Can you work these out from the model? Positions are in its coordinate system, mm. Face numbers are marked on the shaded views. A direction names the side the tool comes from. Round coordinates to 2 decimals unless told otherwise and drop trailing zeros. Write each loop counter-clockwise with the first axis right and the second up, starting at its lowest first coordinate (ties: lowest second). Pieces come first, ordered by that corner, then holes. Notation, with made-up numbers: M 1,4 L 13,4 A34 ccw 13,36 Z; hole C -27,42.5 d9. An arc over 180 degrees is marked long. Answer in a Markdown table with one row per item. Add a question column.
(1) Suppose I cut it at A-A, the plane x = 2.5. Write out the boundary of the cut face in (y, z), then the cut area to 3 significant figures.
(2) I'm going to push flat-ended pins straight in: pin 1 (3 mm diameter, centred on y = -5, z = 4.5, fed in from +X); pin 2 (3 mm diameter, centred on x = 0, y = 0, fed in from +Z); pin 3 (3 mm diameter, centred on y = 7, z = 4.5, fed in from +X). Where does each tip first touch, or does it pass through?
(3) If we mould it in two halves opening along Y, with no side actions, what happens to the marked faces 5, 6 and 7? For each: released by +Y, released by -Y, zero draft, split by the parting line, or undercut.
(4) If I drill on probe 1 along Y at (x, z) = (0, 7.4); probe 2 along Y at (x, z) = (-12, 7); probe 3 along X at (y, z) = (10.25, 6), over which ranges is the centre line in solid material (lowest first)?
(5) Suppose I cut it at B-B, the plane x = -8.75. Write out the boundary of the cut face in (y, z), then the cut area to 3 significant figures.
(6) For the marked faces 1, 2, 3 and 4, which set-ups out of +Z, -Z, +X, -X, +Y, -Y let a thin tool reach every point of the face, with its end or its side?
(7) Suppose I cut it at C-C, the plane x = 9. Write out the boundary of the cut face in (y, z).
from build123d import *

# Parameters (mm, degrees)
BOSS_EXTRUDE1_DEPTH = 7.6
SKETCH4_R           = 1.75
CUT_EXTRUDE1_DEPTH  = 7
SKETCH5_R           = 1.75
CUT_EXTRUDE2_DEPTH  = 21.680425528


with BuildPart() as part:
    # Sketch1 → Boss-Extrude1 (new body)
    with BuildSketch(Plane.XY):
        with BuildLine():
            Line((-0.124457167, 13.6), (0.124457167, 13.6))
            ThreePointArc((0.124457167, 13.6), (0.424734881, 13.499791564), (0.604651154, 13.23933318))
            Line((0.604651154, 13.23933318), (1.275962124, 10.925745771))
            ThreePointArc((1.275962124, 10.925745771), (1.720779115, 10.864571747), (2.162729027, 10.785295692))
            Line((2.162729027, 10.785295692), (3.516121527, 12.778201575))
            ThreePointArc((3.516121527, 12.778201575), (3.767718138, 12.970315032), (4.084265323, 12.972828001))
            Line((4.084265323, 12.972828001), (4.320996924, 12.895909242))
            ThreePointArc((4.320996924, 12.895909242), (4.57561189, 12.70781444), (4.666236367, 12.40450661))
            Line((4.666236367, 12.40450661), (4.589753212, 9.996707731))
            ThreePointArc((4.589753212, 9.996707731), (4.993895497, 9.801071766), (5.389717192, 9.589105724))
            Line((5.389717192, 9.589105724), (7.292711734, 11.066250568))
            ThreePointArc((7.292711734, 11.066250568), (7.591360654, 11.171213695), (7.893191468, 11.075785211))
            Line((7.893191468, 11.075785211), (8.094567395, 10.929477036))
            ThreePointArc((8.094567395, 10.929477036), (8.278596127, 10.671907897), (8.271057853, 10.355440506))
            Line((8.271057853, 10.355440506), (7.454267277, 8.089122286))
            ThreePointArc((7.454267277, 8.089122286), (7.778174593, 7.778174593), (8.089122286, 7.454267277))
            Line((8.089122286, 7.454267277), (10.355440506, 8.271057853))
            ThreePointArc((10.355440506, 8.271057853), (10.671907897, 8.278596127), (10.929477036, 8.094567395))
            Line((10.929477036, 8.094567395), (11.075785211, 7.893191468))
            ThreePointArc((11.075785211, 7.893191468), (11.171213695, 7.591360654), (11.066250568, 7.292711734))
            Line((11.066250568, 7.292711734), (9.589105724, 5.389717192))
            ThreePointArc((9.589105724, 5.389717192), (9.801071766, 4.993895497), (9.996707731, 4.589753212))
            Line((9.996707731, 4.589753212), (12.40450661, 4.666236367))
            ThreePointArc((12.40450661, 4.666236367), (12.70781444, 4.57561189), (12.895909242, 4.320996924))
            Line((12.895909242, 4.320996924), (12.972828001, 4.084265323))
            ThreePointArc((12.972828001, 4.084265323), (12.970315032, 3.767718138), (12.778201575, 3.516121527))
            Line((12.778201575, 3.516121527), (10.785295692, 2.162729027))
            ThreePointArc((10.785295692, 2.162729027), (10.864571747, 1.720779115), (10.925745771, 1.275962124))
            Line((10.925745771, 1.275962124), (13.23933318, 0.604651154))
            ThreePointArc((13.23933318, 0.604651154), (13.499791564, 0.424734881), (13.6, 0.124457167))
            Line((13.6, 0.124457167), (13.6, -0.124457167))
            ThreePointArc((13.6, -0.124457167), (13.499791564, -0.424734881), (13.23933318, -0.604651154))
            Line((13.23933318, -0.604651154), (10.925745771, -1.275962124))
            ThreePointArc((10.925745771, -1.275962124), (10.864571747, -1.720779115), (10.785295692, -2.162729027))
            Line((10.785295692, -2.162729027), (12.778201575, -3.516121527))
            ThreePointArc((12.778201575, -3.516121527), (12.970315032, -3.767718138), (12.972828001, -4.084265323))
            Line((12.972828001, -4.084265323), (12.895909242, -4.320996924))
            ThreePointArc((12.895909242, -4.320996924), (12.70781444, -4.57561189), (12.40450661, -4.666236367))
            Line((12.40450661, -4.666236367), (9.996707731, -4.589753212))
            ThreePointArc((9.996707731, -4.589753212), (9.801071766, -4.993895497), (9.589105724, -5.389717192))
            Line((9.589105724, -5.389717192), (11.066250568, -7.292711734))
            ThreePointArc((11.066250568, -7.292711734), (11.171213695, -7.591360654), (11.075785211, -7.893191468))
            Line((11.075785211, -7.893191468), (10.929477036, -8.094567395))
            ThreePointArc((10.929477036, -8.094567395), (10.671907897, -8.278596127), (10.355440506, -8.271057853))
            Line((10.355440506, -8.271057853), (8.089122286, -7.454267277))
            ThreePointArc((8.089122286, -7.454267277), (7.778174593, -7.778174593), (7.454267277, -8.089122286))
            Line((7.454267277, -8.089122286), (8.271057853, -10.355440506))
            ThreePointArc((8.271057853, -10.355440506), (8.278596127, -10.671907897), (8.094567395, -10.929477036))
            Line((8.094567395, -10.929477036), (7.893191468, -11.075785211))
            ThreePointArc((7.893191468, -11.075785211), (7.591360654, -11.171213695), (7.292711734, -11.066250568))
            Line((7.292711734, -11.066250568), (5.389717192, -9.589105724))
            ThreePointArc((5.389717192, -9.589105724), (4.993895497, -9.801071766), (4.589753212, -9.996707731))
            Line((4.589753212, -9.996707731), (4.666236367, -12.40450661))
            ThreePointArc((4.666236367, -12.40450661), (4.57561189, -12.70781444), (4.320996924, -12.895909242))
            Line((4.320996924, -12.895909242), (4.084265323, -12.972828001))
            ThreePointArc((4.084265323, -12.972828001), (3.767718138, -12.970315032), (3.516121527, -12.778201575))
            Line((3.516121527, -12.778201575), (2.162729027, -10.785295692))
            ThreePointArc((2.162729027, -10.785295692), (1.720779115, -10.864571747), (1.275962124, -10.925745771))
            Line((1.275962124, -10.925745771), (0.604651154, -13.23933318))
            ThreePointArc((0.604651154, -13.23933318), (0.424734881, -13.499791564), (0.124457167, -13.6))
            Line((0.124457167, -13.6), (-0.124457167, -13.6))
            ThreePointArc((-0.124457167, -13.6), (-0.424734881, -13.499791564), (-0.604651154, -13.23933318))
            Line((-0.604651154, -13.23933318), (-1.275962124, -10.925745771))
            ThreePointArc((-1.275962124, -10.925745771), (-1.720779115, -10.864571747), (-2.162729027, -10.785295692))
            Line((-2.162729027, -10.785295692), (-3.516121527, -12.778201575))
            ThreePointArc((-3.516121527, -12.778201575), (-3.767718138, -12.970315032), (-4.084265323, -12.972828001))
            Line((-4.084265323, -12.972828001), (-4.320996924, -12.895909242))
            ThreePointArc((-4.320996924, -12.895909242), (-4.57561189, -12.70781444), (-4.666236367, -12.40450661))
            Line((-4.666236367, -12.40450661), (-4.589753212, -9.996707731))
            ThreePointArc((-4.589753212, -9.996707731), (-4.993895497, -9.801071766), (-5.389717192, -9.589105724))
            Line((-5.389717192, -9.589105724), (-7.292711734, -11.066250568))
            ThreePointArc((-7.292711734, -11.066250568), (-7.591360654, -11.171213695), (-7.893191468, -11.075785211))
            Line((-7.893191468, -11.075785211), (-8.094567395, -10.929477036))
            ThreePointArc((-8.094567395, -10.929477036), (-8.278596127, -10.671907897), (-8.271057853, -10.355440506))
            Line((-8.271057853, -10.355440506), (-7.454267277, -8.089122286))
            ThreePointArc((-7.454267277, -8.089122286), (-7.778174593, -7.778174593), (-8.089122286, -7.454267277))
            Line((-8.089122286, -7.454267277), (-10.355440506, -8.271057853))
            ThreePointArc((-10.355440506, -8.271057853), (-10.671907897, -8.278596127), (-10.929477036, -8.094567395))
            Line((-10.929477036, -8.094567395), (-11.075785211, -7.893191468))
            ThreePointArc((-11.075785211, -7.893191468), (-11.171213695, -7.591360654), (-11.066250568, -7.292711734))
            Line((-11.066250568, -7.292711734), (-9.589105724, -5.389717192))
            ThreePointArc((-9.589105724, -5.389717192), (-9.801071766, -4.993895497), (-9.996707731, -4.589753212))
            Line((-9.996707731, -4.589753212), (-12.40450661, -4.666236367))
            ThreePointArc((-12.40450661, -4.666236367), (-12.70781444, -4.57561189), (-12.895909242, -4.320996924))
            Line((-12.895909242, -4.320996924), (-12.972828001, -4.084265323))
            ThreePointArc((-12.972828001, -4.084265323), (-12.970315032, -3.767718138), (-12.778201575, -3.516121527))
            Line((-12.778201575, -3.516121527), (-10.785295692, -2.162729027))
            ThreePointArc((-10.785295692, -2.162729027), (-10.864571747, -1.720779115), (-10.925745771, -1.275962124))
            Line((-10.925745771, -1.275962124), (-13.23933318, -0.604651154))
            ThreePointArc((-13.23933318, -0.604651154), (-13.499791564, -0.424734881), (-13.6, -0.124457167))
            Line((-13.6, -0.124457167), (-13.6, 0.124457167))
            ThreePointArc((-13.6, 0.124457167), (-13.499791564, 0.424734881), (-13.23933318, 0.604651154))
            Line((-13.23933318, 0.604651154), (-10.925745771, 1.275962124))
            ThreePointArc((-10.925745771, 1.275962124), (-10.864571747, 1.720779115), (-10.785295692, 2.162729027))
            Line((-10.785295692, 2.162729027), (-12.778201575, 3.516121527))
            ThreePointArc((-12.778201575, 3.516121527), (-12.970315032, 3.767718138), (-12.972828001, 4.084265323))
            Line((-12.972828001, 4.084265323), (-12.895909242, 4.320996924))
            ThreePointArc((-12.895909242, 4.320996924), (-12.70781444, 4.57561189), (-12.40450661, 4.666236367))
            Line((-12.40450661, 4.666236367), (-9.996707731, 4.589753212))
            ThreePointArc((-9.996707731, 4.589753212), (-9.801071766, 4.993895497), (-9.589105724, 5.389717192))
            Line((-9.589105724, 5.389717192), (-11.066250568, 7.292711734))
            ThreePointArc((-11.066250568, 7.292711734), (-11.171213695, 7.591360654), (-11.075785211, 7.893191468))
            Line((-11.075785211, 7.893191468), (-10.929477036, 8.094567395))
            ThreePointArc((-10.929477036, 8.094567395), (-10.671907897, 8.278596127), (-10.355440506, 8.271057853))
            Line((-10.355440506, 8.271057853), (-8.089122286, 7.454267277))
            ThreePointArc((-8.089122286, 7.454267277), (-7.778174593, 7.778174593), (-7.454267277, 8.089122286))
            Line((-7.454267277, 8.089122286), (-8.271057853, 10.355440506))
            ThreePointArc((-8.271057853, 10.355440506), (-8.278596127, 10.671907897), (-8.094567395, 10.929477036))
            Line((-8.094567395, 10.929477036), (-7.893191468, 11.075785211))
            ThreePointArc((-7.893191468, 11.075785211), (-7.591360654, 11.171213695), (-7.292711734, 11.066250568))
            Line((-7.292711734, 11.066250568), (-5.389717192, 9.589105724))
            ThreePointArc((-5.389717192, 9.589105724), (-4.993895497, 9.801071766), (-4.589753212, 9.996707731))
            Line((-4.589753212, 9.996707731), (-4.666236367, 12.40450661))
            ThreePointArc((-4.666236367, 12.40450661), (-4.57561189, 12.70781444), (-4.320996924, 12.895909242))
            Line((-4.320996924, 12.895909242), (-4.084265323, 12.972828001))
            ThreePointArc((-4.084265323, 12.972828001), (-3.767718138, 12.970315032), (-3.516121527, 12.778201575))
            Line((-3.516121527, 12.778201575), (-2.162729027, 10.785295692))
            ThreePointArc((-2.162729027, 10.785295692), (-1.720779115, 10.864571747), (-1.275962124, 10.925745771))
            Line((-1.275962124, 10.925745771), (-0.604651154, 13.23933318))
            ThreePointArc((-0.604651154, 13.23933318), (-0.424734881, 13.499791564), (-0.124457167, 13.6))
        make_face()
    extrude(amount=BOSS_EXTRUDE1_DEPTH)

    # Sketch4 → Cut-Extrude1 (cut)
    with BuildSketch(Plane(origin=(0, 0, 0), x_dir=(-1, 0, 0), z_dir=(0, 0, -1))):
        Polygon((-6.926368188, -0.15944818), (-3.325097919, -6.078134897), (3.601270269, -5.918686717), (6.926368188, 0.15944818), (3.325097919, 6.078134897), (-3.601270269, 5.918686717), align=None)
        Circle(SKETCH4_R, mode=Mode.SUBTRACT)
    extrude(amount=-CUT_EXTRUDE1_DEPTH, mode=Mode.SUBTRACT)

    # Sketch5 → Cut-Extrude2 (cut, through all)
    with BuildSketch(Plane(origin=(0, 0, 0), x_dir=(-1, 0, 0), z_dir=(0, 0, -1))):
        Circle(SKETCH5_R)
    extrude(amount=-CUT_EXTRUDE2_DEPTH, mode=Mode.SUBTRACT)


solid = part.part
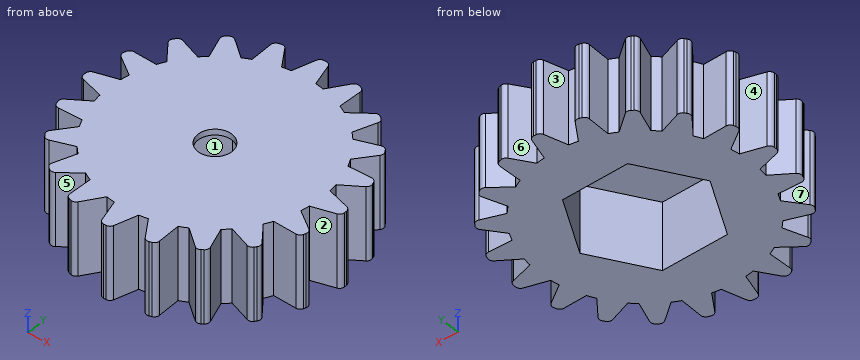
Calculated:
| question | item | result |
|---|---|---|
| 1 | outline | M -11.28,0 L -6.06,0 L -6.06,7 L 5.94,7 L 5.94,0 L 11.28,0 L 11.28,7.6 L -11.28,7.6 Z |
| 1 | area | 87.5 mm² |
| 2 | pin 1 | x = 13 |
| 2 | pin 2 | through |
| 2 | pin 3 | x = 11.17 |
| 3 | face 5 | released by -Y |
| 3 | face 6 | released by +Y |
| 3 | face 7 | undercut |
| 4 | probe 1 | -13.6 to -1.75, 1.75 to 13.6 |
| 4 | probe 2 | -4.65 to -2.99, -0.96 to 0.96, 2.99 to 4.65 |
| 4 | probe 3 | -8.23 to -6.24, -4.6 to 4.6, 6.24 to 8.23 |
| 5 | outline | M -7.69,0 L 7.69,0 L 7.69,7.6 L -7.69,7.6 Z |
| 5 | area | 117 mm² |
| 6 | face 1 | -Z |
| 6 | face 2 | +Z, -Z, +X |
| 6 | face 3 | +Z, -Z, +Y |
| 6 | face 4 | +Z, -Z, -X |
| 7 | outline | M -7.78,0 L 7.78,0 L 7.78,7.6 L -7.78,7.6 Z |
